Here's how the part is built. I have some questions about the finished solid (model axes, mm). A direction names the side the tool comes from. Coordinates: 2 decimals unless noted, no trailing zeros. Write each loop counter-clockwise with the first axis right and the second up, starting at its lowest first coordinate (ties: lowest second). Pieces come first, ordered by that corner, then holes. Notation, with made-up numbers: (62.5, 28) - (74.5, 28) arc R14 ccw to (74.5, 37) - close; hole circle Ø9 at (22.5, 61). An arc over 180 degrees is marked (long way). Answer in a Markdown table with one row per item. Add a question column.
Item 1: I'm going to push flat-ended pins straight in: pin 1 (3 mm diameter, centred on y = -4.5, z = 5, fed in from -X); pin 2 (1 mm diameter, centred on y = 3.5, z = 4.5, fed in from +X). Where does each tip first touch, or does it pass through?
Item 2: If I drill on probe 1 along Y at (x, z) = (-2, 5.75); probe 2 along Y at (x, z) = (1, 2.75); probe 3 along X at (y, z) = (1, 1.75), over which ranges is the centre line in solid material (lowest first)? Write a range as from..to.
Item 3: Imagine slicing it at D-D (x = 8.5). Please give me the cut outline in (y, z), plus the area to 3 significant figures.
Item 4: Imagine slicing it at C-C (y = 7). Please give me the cut outline in (x, z).
Item 5: Which directions (+Z, -Z, +X, -X, +Y, -Y) give clear straight access to the entire face, cutting with the end or side of a thin tool? Please do faces 1 (the face through (-3, 10, 6.35)), 2 (the face through (-7.73, 19.54, 3.13)), 3 (the face through (4.383, 7.365, 3.131)).
Item 6: Imagine slicing it at B-B (x = -2.5). Please give me the cut outline in (y, z).
Item 7: We'd pull the mould along Y, two halves only. Please class faces 4 (the face through (0.048, 18.474, 3.131)), 5 (the face through (-3, 10, 0)), 6 (the face through (4.46, 2.26, 3.13)): +Y half, -Y half, draft (parallel to the pull), parting line (faces both ways), or undercut.
Item 8: Imagine slicing it at A-A (z = 5.5). Please give me the cut outline in (x, y).
from build123d import *

# Parameters (mm, degrees)
F1_DEPTH = 6.35


with BuildPart() as f1:
    # F0 (on Top) → F1 (new body)
    with BuildSketch(Plane.XY):
        with BuildLine():
            Line((-12.188626, 21.072123), (-12.047861, 11.32767))
            ThreePointArc((-12.047861, 11.32767), (0, -8.98224), (12.047861, 11.32767))
            Line((12.047861, 11.32767), (12.188626, 21.072123))
            Line((12.188626, 21.072123), (3.397549, 18.047413))
            ThreePointArc((3.397549, 18.047413), (0, 18.474475), (-3.397549, 18.047413))
            Line((-3.397549, 18.047413), (-12.188626, 21.072123))
        make_face()
        Polygon((-2.982468, 9.831229), (2.912602, 9.871567), (5.89507, 4.786455), (2.982468, -0.338994), (-2.912602, -0.379331), (-5.89507, 4.70578), align=None, mode=Mode.SUBTRACT)
    extrude(amount=F1_DEPTH)


solid = f1.part
Here are the results:
| question | item | result |
|---|---|---|
| 1 | pin 1 | stops at x = -11.33 |
| 1 | pin 2 | stops at x = 13.71 |
| 2 | probe 1 | y = -8.84..-0.37, 9.84..18.33 |
| 2 | probe 2 | y = -8.95..-0.35, 9.86..18.44 |
| 2 | probe 3 | x = -13.21..-3.72, 3.74..13.21 |
| 3 | outline | (-6.03, 0) - (19.8, 0) - (19.8, 6.35) - (-6.03, 6.35) - close |
| 3 | area | 164 mm2 |
| 4 | outline | (-13.54, 0) - (-4.59, 0) - (-4.59, 6.35) - (-13.54, 6.35) - close; (4.6, 0) - (13.54, 0) - (13.54, 6.35) - (4.6, 6.35) - close |
| 5 | face 1 | +Z, +X, -X, +Y, -Y |
| 5 | face 2 | +Z, -Z, +Y |
| 5 | face 3 | +Z, -Z |
| 6 | outline | (-8.75, 0) - (-0.38, 0) - (-0.38, 6.35) - (-8.75, 6.35) - close; (9.83, 0) - (18.24, 0) - (18.24, 6.35) - (9.83, 6.35) - close |
| 7 | face 4 | +Y half |
| 7 | face 5 | draft |
| 7 | face 6 | undercut |
| 8 | outline | (-12.19, 21.07) - (-12.05, 11.33) arc R13.73 ccw (long way) to (12.05, 11.33) - (12.19, 21.07) - (3.4, 18.05) arc R13.73 ccw to (-3.4, 18.05) - close; hole (-5.9, 4.71) - (-2.91, -0.38) - (2.98, -0.34) - (5.9, 4.79) - (2.91, 9.87) - (-2.98, 9.83) - close |
